Study the drawing (mm; zero at the part's minimum x, y, z) and answer. A direction names the side the tool comes from. Give positions to 0.01 mm unless a question says otherwise; leave off trailing zeros. Write each loop counter-clockwise with the first axis right and the second up, starting at its lowest first coordinate (ties: lowest second). Pieces come first, ordered by that corner, then holes. Notation, with made-up numbers: (66, 47.25) -> (89, 47.25) arc R25 cw to (89, 79.25) -> close; hole circle Ø9 at (55, 79.25). An arc over 180 degrees is marked (long way). One line per question, with ' | ' between items.
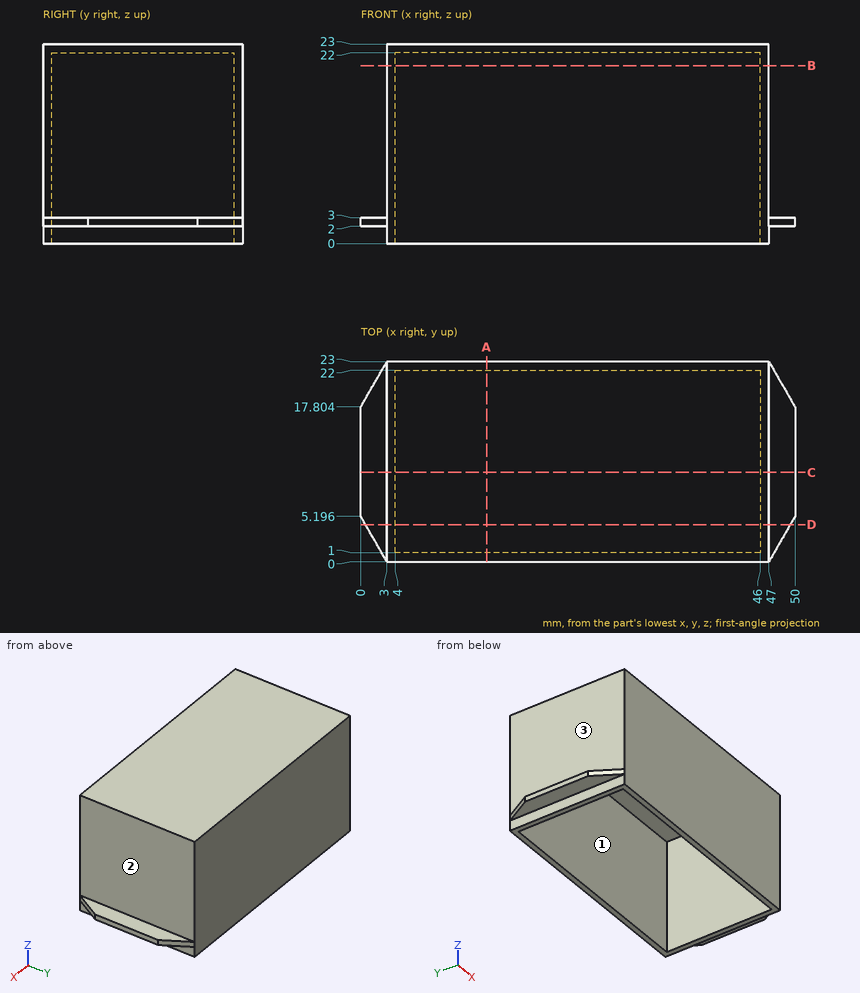
Item 1: Find section B-B (z = 20.5). Write down the section's boundary in (x, y).
Answers below:
outline: (3, 0) -> (47, 0) -> (47, 23) -> (3, 23) -> close; hole (4, 1) -> (46, 1) -> (46, 22) -> (4, 22) -> close
Item 2: A tool of negligible diameter and unlimited length cuts with its end or side. For the marked faces 1, 2 and 3, from which of +Z, -Z, +X, -X, +Y, -Y can it reach the whole face along a straight path? Write none if from no direction.
Answers below:
face 1: -Z | face 2: +Z, +X, +Y, -Y | face 3: +Z, -X, +Y, -Y
Item 3: Find section A-A (x = 14.5). Write down the section's boundary in (y, z).
Answers below:
outline: (0, 0) -> (1, 0) -> (1, 22) -> (22, 22) -> (22, 0) -> (23, 0) -> (23, 23) -> (0, 23) -> close
Item 4: Consider line 1 (X direction, y = 8.5, z = 5); line 2 (Y direction, x = 45.5, z = 14); line 3 (X direction, y = 6.25, z = 2.5). Determine where each line is inside the solid, lowest interval first. Write a range as [from, to].
Answers below:
line 1: [3, 4], [46, 47] | line 2: [0, 1], [22, 23] | line 3: [0, 4], [46, 50]
Item 5: Find section D-D (y = 4.25). Write down the section's boundary in (x, z).
Answers below:
outline: (0.55, 2) -> (3, 2) -> (3, 0) -> (4, 0) -> (4, 22) -> (46, 22) -> (46, 0) -> (47, 0) -> (47, 2) -> (49.45, 2) -> (49.45, 3) -> (47, 3) -> (47, 23) -> (3, 23) -> (3, 3) -> (0.55, 3) -> close
Item 6: Flat-ended cylindrical pins translate along their axes: pin 1 (1.5 mm diameter, centred on x = 48.5, y = 11.5, fed in from +Z); pin 2 (1.5 mm diameter, centred on y = 14, z = 17.5, fed in from -X); pin 3 (0.9 mm diameter, centred on x = 1, y = 8.5, fed in from -Z). Find the tip coordinate at first contact, or state that the pin passes through.
Answers below:
pin 1: z = 3 | pin 2: x = 3 | pin 3: z = 2
Item 7: Find section C-C (y = 10.25). Write down the section's boundary in (x, z).
Answers below:
outline: (0, 2) -> (3, 2) -> (3, 0) -> (4, 0) -> (4, 22) -> (46, 22) -> (46, 0) -> (47, 0) -> (47, 2) -> (50, 2) -> (50, 3) -> (47, 3) -> (47, 23) -> (3, 23) -> (3, 3) -> (0, 3) -> close
